Geometry check sheet. Reference: the model listing, model coordinates, mm. A direction names the side the tool comes from. Round coordinates to 2 decimals unless told otherwise and drop trailing zeros. Write each loop counter-clockwise with the first axis right and the second up, starting at its lowest first coordinate (ties: lowest second). Pieces come first, ordered by that corner, then holes. Notation, with made-up numbers: M 71.25,4 L 129.25,4 A31 ccw 129.25,43 Z; hole C 47.25,72 d10. An arc over 180 degrees is marked long. One line per item, written item: value. Start each with the question number.
1. Depth check by flat-ended pin: P1, Ø2, axis at x = 84, y = 44.5, coming from the -Z side; P2, Ø3, axis at y = 45, z = -3.5, coming from the +X side; P3, Ø3, axis at x = 78.5, z = -1, coming from the +Y side; P4, Ø2, axis at x = 82, z = 0, coming from the -Y side. Enter the tip coordinate at first touch or a pass-through.
2. Section check B-B (x = 82.75). Record the boundary of the cut face in (y, z), and give its area (4 significant figures).
3. Section check C-C (z = 1.5). Record the boundary of the cut face in (x, y), and give its area (3 significant figures).
4. Release check for a two-part mould opening along Y. For faces 4 (the cylindrical face through (81.65, 45.15, 2.84)), 5 (the cylindrical face through (85.17, 40.54, -4.01)), 6 (the flat face through (84, 44, 3.7)) record: pulls with the +Y half, pulls with the -Y half, needs draft (parallel to the pull), parting line crosses it, or undercut.
5. Scan lines: probe 1 along Y at (x, z) = (82.75, -1); probe 2 along Y at (x, z) = (82.75, 2.9); probe 3 along Z at (x, y) = (82.25, 40.5). Record each from-to range of solid material in increasing order. Write a range as [from, to].
6. Access from +Z, -Z, +X, -X, +Y, -Y to the whole of each face (thin tool, end or side, straight path). Record for faces 1 (the flat face through (82, 44, 2)), 2 (the cylindrical face through (82.249, 49.017, 0.303)), 3 (the flat face through (86.2, 46.4, -5)).
7. Section check A-A (y = 45.2). Record the boundary of the cut face in (x, z).
8. Section check D-D (x = 86). Record the boundary of the cut face in (y, z), and give its area (3 significant figures).
from build123d import *

# Parameters (mm, degrees)
SKETCH111_R     = 5.25
PAD063_DEPTH    = 2
SKETCH112_R     = 3.85
PAD064_DEPTH    = 6.7
SKETCH113_R     = 3.5
POCKET047_DEPTH = 7
SKETCH114_R     = 1.1
POCKET048_DEPTH = 5


with BuildPart() as part:
    # Sketch111 → Pad063 (new body)
    with BuildSketch(Plane.XY):
        Circle(SKETCH111_R)
    extrude(amount=PAD063_DEPTH)

    # Sketch112 (on Face3 of Pad063) → Pad064 (join)
    with BuildSketch(Plane.XY.offset(2)):
        Circle(SKETCH112_R)
    extrude(amount=PAD064_DEPTH)

    # Sketch113 (on Face2 of Pad064) → Pocket047 (cut)
    with BuildSketch(Plane(origin=(0, 0, 0), x_dir=(1, 0, 0), z_dir=(0, 0, -1))):
        Circle(SKETCH113_R)
    extrude(amount=-POCKET047_DEPTH, mode=Mode.SUBTRACT)

    # Sketch114 (on Face6 of Pocket047) → Pocket048 (cut)
    with BuildSketch(Plane(origin=(0, 0, 7), x_dir=(1, 0, 0), z_dir=(0, 0, -1))):
        Circle(SKETCH114_R)
    extrude(amount=-POCKET048_DEPTH, mode=Mode.SUBTRACT)


with BuildPart() as part_1:
    # Body022 placement: moved
    add(part.part.moved(Location((82.75, 45.2, -5))))


solid = part_1.part
Result sheet:
1. P1: stops at z = 2
1. P2: stops at x = 88
1. P3: stops at y = 47.89
1. P4: stops at y = 41.35
2. outline: M 39.95,-5 L 41.7,-5 L 41.7,2 L 44.1,2 L 44.1,3.7 L 41.35,3.7 L 41.35,-3 L 39.95,-3 Z; M 46.3,2 L 48.7,2 L 48.7,-5 L 50.45,-5 L 50.45,-3 L 49.05,-3 L 49.05,3.7 L 46.3,3.7 Z
2. area: 19.85 mm2
3. outline: C 82.75,45.2 d7.7; hole C 82.75,45.2 d7
3. area: 8.08 mm2
4. face 4: undercut
4. face 5: parting line crosses it
4. face 6: needs draft
5. probe 1: y = [41.35, 41.7], [48.7, 49.05]
5. probe 2: y = [41.35, 44.1], [46.3, 49.05]
5. probe 3: z = [-5, -3]
6. face 1: -Z
6. face 2: +Z
6. face 3: -Z, +X, -X, +Y, -Y
7. outline: M 77.5,-5 L 79.25,-5 L 79.25,2 L 81.65,2 L 81.65,3.7 L 78.9,3.7 L 78.9,-3 L 77.5,-3 Z; M 83.85,2 L 86.25,2 L 86.25,-5 L 88,-5 L 88,-3 L 86.6,-3 L 86.6,3.7 L 83.85,3.7 Z
8. outline: M 41.08,-5 L 43.9,-5 L 43.9,2 L 46.5,2 L 46.5,-5 L 49.32,-5 L 49.32,-3 L 47.26,-3 L 47.26,3.7 L 43.14,3.7 L 43.14,-3 L 41.08,-3 Z
8. area: 26.0 mm2
